Can you work these out from the drawing? Everything is in mm from the part's minimum corner. A direction names the side the tool comes from. Give positions to 0.01 mm unless a question says otherwise; leave off trailing zeros. Loops run counter-clockwise (first coordinate to the right, second up) from the corner with the lowest first, then second, coordinate; pieces in that order, holes last. Notation, with made-up numbers: (63, 53.5) - (89, 53.5) arc R23 ccw to (89, 71.5) - close; hole circle Ø10 at (13, 29.25). An arc over 180 degrees is marked (long way). Answer in a Markdown table with one row per item. Add a question column.
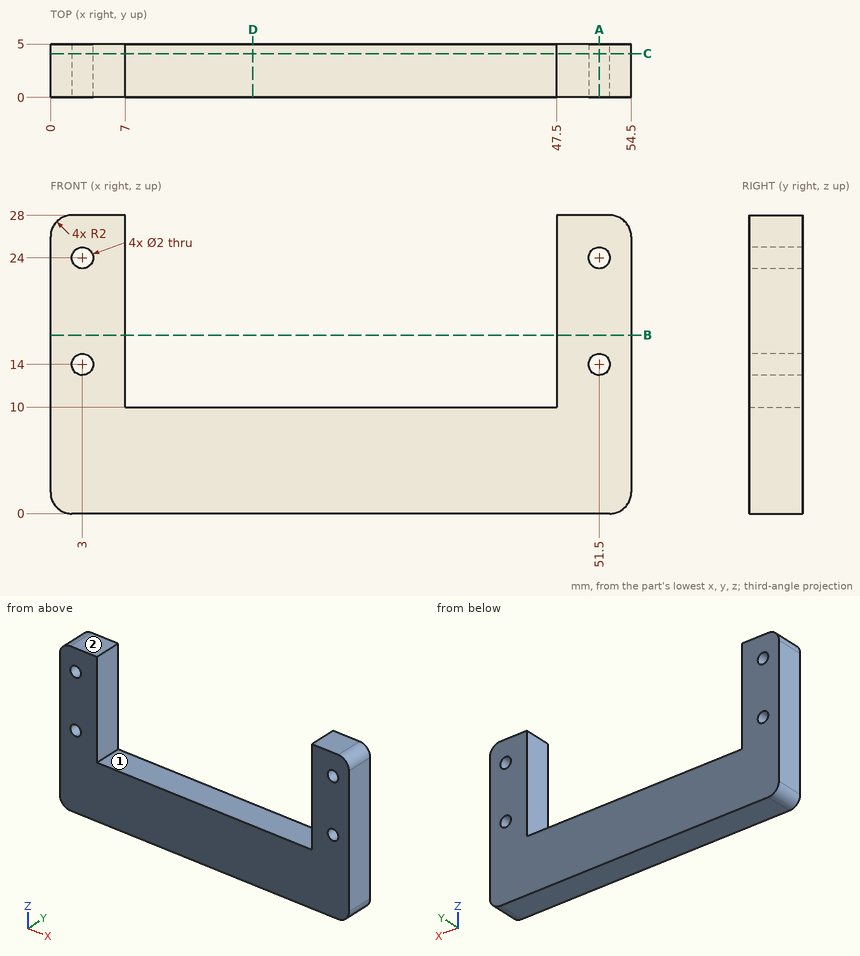
(1) I want a section at A-A on x = 51.5. Please give me the cut outline in (y, z).
(2) Please list where these lines run through material, in increasing order: line 1 (X direction, y = 1.25, z = 14); line 2 (Z direction, x = 3, y = 3.2); line 3 (X direction, y = 1.05, z = 20.5).
(3) For pin 1 Ø1 at (x, y) = (9.5, 2.5) entering from +Z, with a flat end and sliding along its axis, tell me the tip position at first contact or that it passes through.
(4) I want a section at D-D on x = 19. Please give me the cut outline in (y, z).
(5) I want a section at B-B on z = 16.75. Please give me the cut outline in (x, y).
(6) I want a section at C-C on y = 4.1. Please give me the cut outline in (x, z).
(7) On a 3-axis mill with a long thin cutter (end or side, diameter ignored), from which of +Z, -Z, +X, -X, +Y, -Y can I reach the whole of each face in a straight line? I mean the marked faces 1 and 2. Say none if no direction works.
Reported:
| question | item | result |
|---|---|---|
| 1 | outline | (0, 0) - (5, 0) - (5, 13) - (0, 13) - close; (0, 15) - (5, 15) - (5, 23) - (0, 23) - close; (0, 25) - (5, 25) - (5, 28) - (0, 28) - close |
| 2 | line 1 | 0 to 2, 4 to 7, 47.5 to 50.5, 52.5 to 54.5 |
| 2 | line 2 | 0 to 13, 15 to 23, 25 to 28 |
| 2 | line 3 | 0 to 7, 47.5 to 54.5 |
| 3 | pin 1 | z = 10 |
| 4 | outline | (0, 0) - (5, 0) - (5, 10) - (0, 10) - close |
| 5 | outline | (0, 0) - (7, 0) - (7, 5) - (0, 5) - close; (47.5, 0) - (54.5, 0) - (54.5, 5) - (47.5, 5) - close |
| 6 | outline | (0, 2) arc R2 ccw to (2, 0) - (52.5, 0) arc R2 ccw to (54.5, 2) - (54.5, 26) arc R2 ccw to (52.5, 28) - (47.5, 28) - (47.5, 10) - (7, 10) - (7, 28) - (2, 28) arc R2 ccw to (0, 26) - close; hole circle Ø2 at (3, 14); hole circle Ø2 at (3, 24); hole circle Ø2 at (51.5, 14); hole circle Ø2 at (51.5, 24) |
| 7 | face 1 | +Z, +Y, -Y |
| 7 | face 2 | +Z, +X, -X, +Y, -Y |
